Verification items for the finished model (mm, model axes). A direction names the side the tool comes from. Coordinates: 2 decimals unless noted, no trailing zeros. Order: outer loops, then holes, each group sorted by start corner. A loop starts at its lowest first (then second) coordinate and runs counter-clockwise, first axis right, second up. Notation, with made-up numbers: M 84.25,68 L 103.25,68 A24 cw 103.25,78 Z; hole C 53,57 d11. An arc over 180 degrees is marked long. Answer as a JSON object with one key per item and string values. Group by question number.
(1) Mould release check, pull along X, two halves, no side actions. Record for faces 1 (the face through (27.06, -74.19, -126.75)), 2 (the face through (395, -10, -127)), 3 (the face through (196, -100, -127)): released by +X, released by -X, zero draft, split by the parting line, or undercut.
(2) Access from +Z, -Z, +X, -X, +Y, -Y to the whole of each face (thin tool, end or side, straight path). Record for faces 4 (the face through (0, -10, -127)), 5 (the face through (392, -8, -127)).
(3) Cross-section at B-B (z = -60). Enter the section's corners in (x, y), plus the area to 3 significant figures.
(4) Gauge pin test, flat ends, axial feed: pin 1 Ø4 at (y, z) = (-48.5, -73.5) entering from +X; pin 2 Ø5 at (y, z) = (-9.5, -63.5) entering from -X; pin 3 Ø3 at (x, z) = (263, -37.5) entering from +Y; pin 4 Ø1 at (y, z) = (-88.5, -140) entering from -X. Record the tip position at first contact, or that the pin passes through.
(5) Cross-section at A-A (y = -51). Enter the section's corners in (x, z).
(6) Cross-section at C-C (y = -27). Enter the section's corners in (x, z), plus the area to 3 significant figures.
(7) Cross-section at D-D (x = 299.5). Enter the section's corners in (y, z).
(8) Material ranges on line 1 (X direction, y = -10, z = -152.5); line 2 (Y direction, x = 146.5, z = -192); line 3 (Y direction, x = 315, z = -85), recorded low to high.
from build123d import *


with BuildPart() as part:
    # Sweep1: sweep along a path in Sketch1
    with BuildLine(Plane(origin=(0, 0, 0), x_dir=(1, 0, 0), z_dir=(0, 1, 0))) as sweep1_path:
        Line((197.5, 0), (197.5, 250))
    # Sketch4 → Sweep1 (sweep)
    with BuildSketch(Plane.XY):
        with BuildLine():
            Line((0, 0), (0, -20))
            ThreePointArc((0, -20), (23.431457505, -76.568542495), (80, -100))
            Line((80, -100), (315, -100))
            ThreePointArc((315, -100), (371.568542495, -76.568542495), (395, -20))
            Line((395, -20), (395, 0))
            Line((395, 0), (392, 0))
            Line((392, 0), (392, -17))
            ThreePointArc((392, -17), (368.568542495, -73.568542495), (312, -97))
            Line((312, -97), (83, -97))
            ThreePointArc((83, -97), (26.431457505, -73.568542495), (3, -17))
            Line((3, -17), (3, 0))
            Line((3, 0), (0, 0))
        make_face()
    sweep(path=sweep1_path.line)


solid = part.part
Taken from the geometry:
{
 "1": {"face 1": "undercut", "face 2": "released by +X", "face 3": "zero draft"},
 "2": {"face 4": "+Z, -Z, -X, +Y, -Y", "face 5": "+Z, -Z, +Y"},
 "3": {"outline": "M 0,-20 A80 ccw 80,-100 L 315,-100 A80 ccw 395,-20 L 395,0 L 392,0 L 392,-17 A80 cw 312,-97 L 83,-97 A80 cw 3,-17 L 3,0 L 0,0 Z", "area": "1,770 mm²"},
 "4": {"pin 1": "stops at x = 390.48", "pin 2": "stops at x = 0", "pin 3": "stops at y = -97", "pin 4": "stops at x = 37.86"},
 "5": {"outline": "M 6.25,-250 L 10.58,-250 L 10.58,0 L 6.25,0 Z; M 384.42,-250 L 388.75,-250 L 388.75,0 L 384.42,0 Z"},
 "6": {"outline": "M 0.31,-250 L 3.63,-250 L 3.63,0 L 0.31,0 Z; M 391.37,-250 L 394.69,-250 L 394.69,0 L 391.37,0 Z", "area": "1,660 mm²"},
 "7": {"outline": "M -100,-250 L -97,-250 L -97,0 L -100,0 Z"},
 "8": {"line 1": "x = 0 to 3, 392 to 395", "line 2": "y = -100 to -97", "line 3": "y = -100 to -96.94"}
}
